Can you work these out from the model? Positions are in its coordinate system, mm. A direction names the side the tool comes from. Give positions to 0.01 mm unless a question says otherwise; leave off trailing zeros. Order: outer loops, then holes, each group sorted by start corner. A loop starts at its lowest first (then second) coordinate and runs counter-clockwise, first axis right, second up. Notation, with made-up numbers: (-28, -7) -> (23, -7) arc R17 ccw to (23, -1) -> close; hole circle Ø4 at (83.5, -1). An arc over 180 degrees is marked (long way). Answer as a JSON object with one key per item and string values.
```python
from build123d import *

# Parameters (mm, degrees)
CHAFL_N1_SIZE = 1.5
REDONDEO1_R   = 0.5


with BuildPart() as part:
    # Croquis1 → Revolución1 (revolve)
    with BuildSketch(Plane.XY):
        Polygon((0, -22.5), (7, -22.5), (7, -18.5), (9, -18.5), (9, -15.5), (7, -15.5), (7, 9.5), (3.75, 9.5), (3.75, 13.5), (7, 13.5), (7, 22.5), (0, 22.5), align=None)
    revolve(axis=Axis((0, 22.5, 0), (0, -1, 0)))

    # Chaflán1
    chafl_n1_edges = [part.edges().sort_by_distance(p)[0] for p in [
        (-7, 22.5, 0),
    ]]
    chamfer(chafl_n1_edges, length=CHAFL_N1_SIZE)

    # Redondeo1
    redondeo1_edges = [part.edges().sort_by_distance(p)[0] for p in [
        (-7, -22.5, 0),
    ]]
    fillet(redondeo1_edges, radius=REDONDEO1_R)


solid = part.part
```
1. For faces 1 (the face through (6.466, -2.825, -2.681)), 2 (the face through (6.466, -20.226, -2.681)), 3 (the face through (-3, 13.5, -3)), 4 (the face through (-1.172, -16.979, 8.923)), 5 (the face through (0, 22.5, 0)), which set-ups out of +Z, -Z, +X, -X, +Y, -Y let a thin tool reach every point of the face, with its end or its side?
Worked answers:
{"face 1": "+Y", "face 2": "-Y", "face 3": "none", "face 4": "+Y, -Y", "face 5": "+Z, -Z, +X, -X, +Y"}
2. If we section it at C-C on y = -5: Please give me the cut outline in (x, z), then the cut area to 3 significant figures.
Worked answers:
{"outline": "circle Ø14 at (0, 0)", "area": "154 mm²"}
3. If we section it at B-B on z = 0: Please give me the cut outline in (x, y), then the cut area to 3 significant figures.
Worked answers:
{"outline": "(-9, -18.5) -> (-7, -18.5) -> (-7, -22) arc R0.5 ccw to (-6.5, -22.5) -> (6.5, -22.5) arc R0.5 ccw to (7, -22) -> (7, -18.5) -> (9, -18.5) -> (9, -15.5) -> (7, -15.5) -> (7, 9.5) -> (3.75, 9.5) -> (3.75, 13.5) -> (7, 13.5) -> (7, 21) -> (5.5, 22.5) -> (-5.5, 22.5) -> (-7, 21) -> (-7, 13.5) -> (-3.75, 13.5) -> (-3.75, 9.5) -> (-7, 9.5) -> (-7, -15.5) -> (-9, -15.5) -> close", "area": "614 mm²"}
4. If we section it at A-A on x = 0: Please give me the cut outline in (y, z).
Worked answers:
{"outline": "(-22.5, -6.5) arc R0.5 ccw to (-22, -7) -> (-18.5, -7) -> (-18.5, -9) -> (-15.5, -9) -> (-15.5, -7) -> (9.5, -7) -> (9.5, -3.75) -> (13.5, -3.75) -> (13.5, -7) -> (21, -7) -> (22.5, -5.5) -> (22.5, 5.5) -> (21, 7) -> (13.5, 7) -> (13.5, 3.75) -> (9.5, 3.75) -> (9.5, 7) -> (-15.5, 7) -> (-15.5, 9) -> (-18.5, 9) -> (-18.5, 7) -> (-22, 7) arc R0.5 ccw to (-22.5, 6.5) -> close"}
5. If we mould it in two halves opening along Y, with no side actions, what happens to faces 6 (the face through (0, -18.5, -7.3)), 7 (the face through (3, 9.5, -3)), 8 (the face through (0, -15.5, -7.3))? For each: +Y half, -Y half, draft (parallel to the pull), parting line (faces both ways), or undercut.
Worked answers:
{"face 6": "-Y half", "face 7": "undercut", "face 8": "+Y half"}
6. Will these pins go through, and if not, where does the flat tip stop? pin 1 Ø8 at (x, y) = (-4.5, -13) entering from -Z; pin 2 Ø5 at (x, y) = (1.5, 9) entering from +Z.
Worked answers:
{"pin 1": "z = -8.89", "pin 2": "z = 7"}
7. If we section it at D-D on y = 10: Please give me the cut outline in (x, z), then the cut area to 3 significant figures.
Worked answers:
{"outline": "circle Ø7.5 at (0, 0)", "area": "44.2 mm²"}
8. Please list where these lines run through material, in increasing order: L1, parallel to Y at x = -3.5, z = -1.5; L2, parallel to Y at x = -4, z = -7.25; L3, parallel to Y at x = -5.25, z = -4.25.
Worked answers:
{"L1": "-22.5 to 9.5, 13.5 to 22.5", "L2": "-18.5 to -15.5", "L3": "-22.43 to 9.5, 13.5 to 21.25"}
